Source: three-view drawing plus pictorial views. Frame: mm from the lowest corner of the part. Give positions to 0.01 mm unless a question says otherwise; leave off trailing zeros. Loops run counter-clockwise (first coordinate to the right, second up) from the corner with the lowest first, then second, coordinate; pieces in that order, holes last. Notation, with made-up numbers: (18.25, 34) - (30.25, 34) arc R14 cw to (30.25, 46) - close; hole circle Ø11 at (52.25, 87.5). An arc over 180 degrees is marked (long way). Answer as a JSON object with one key per item and string values. Group by question number.
(1) Section query A-A (z = 82.55). Return loops of the section in (x, y).
(2) Section query D-D (z = 31.5). Return loops of the section in (x, y), plus the area to 3 significant figures.
(3) Material intervals for L1, parallel to Z at x = 66, y = 0.2 (1 decimal); L2, parallel to Z at x = 26, y = 3.2 (1 decimal); L3, parallel to X at y = 1.9, z = 55, sorted ascending.
(4) Section query C-C (x = 92). Return loops of the section in (y, z) (1 decimal).
(5) Pin query (flat end, axial travel): P1, Ø1.5, axis at y = 1.5, z = 24.5, coming from the +X side; P2, Ø1, axis at y = 2.5, z = 74, coming from the -X side; P3, Ø1, axis at x = 41, y = 2, coming from the +Z side. Return the tip coordinate at first contact, or that it passes through.
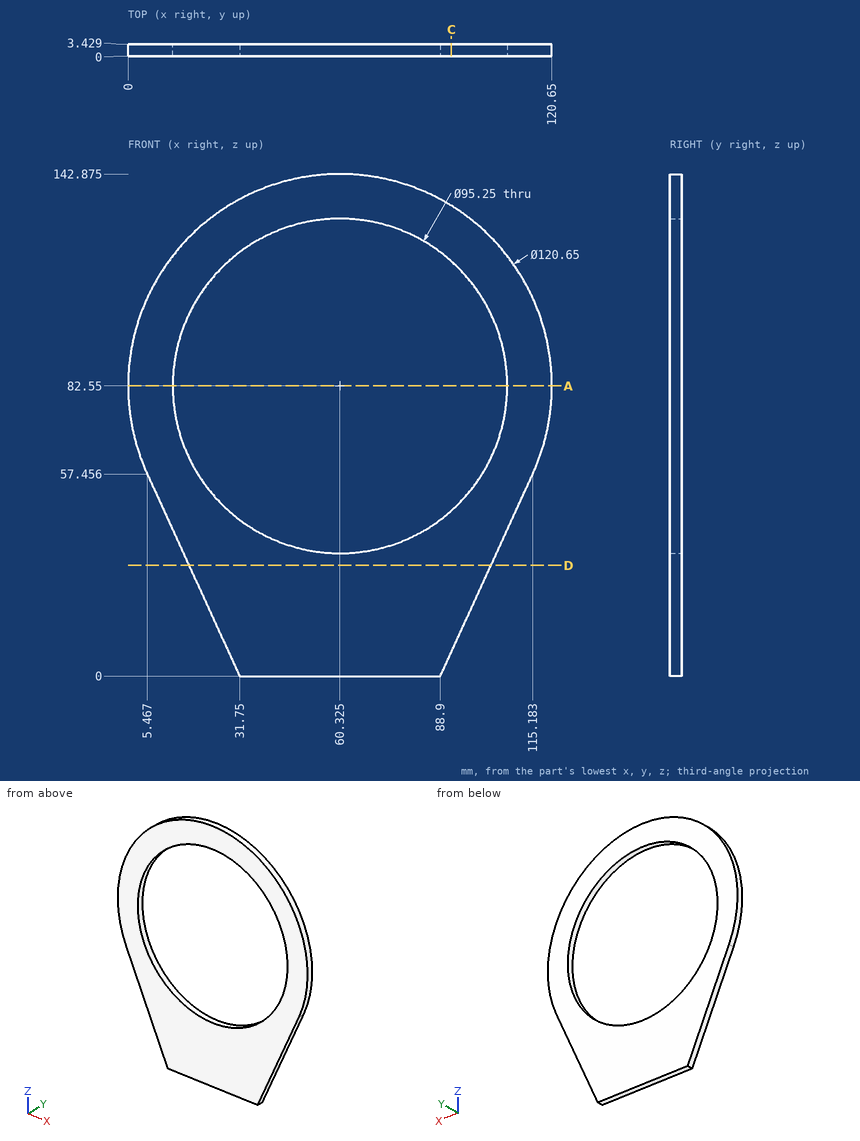
Recorded:
{
 "1": {"outline": "(0, 0) - (12.7, 0) - (12.7, 3.43) - (0, 3.43) - close; (107.95, 0) - (120.65, 0) - (120.65, 3.43) - (107.95, 3.43) - close"},
 "2": {"outline": "(17.34, 0) - (103.31, 0) - (103.31, 3.43) - (17.34, 3.43) - close", "area": "295 mm^2"},
 "3": {"L1": "z = 0 to 35.3, 129.8 to 142.6", "L2": "z = 12.6 to 49.5, 115.6 to 132.2", "L3": "x = 6.59 to 21.48, 99.17 to 114.06"},
 "4": {"outline": "(0, 6.8) - (3.4, 6.8) - (3.4, 47) - (0, 47) - close; (0, 118.1) - (3.4, 118.1) - (3.4, 133.9) - (0, 133.9) - close"},
 "5": {"P1": "stops at x = 100.45", "P2": "stops at x = 0.54", "P3": "stops at z = 139.86"}
}
